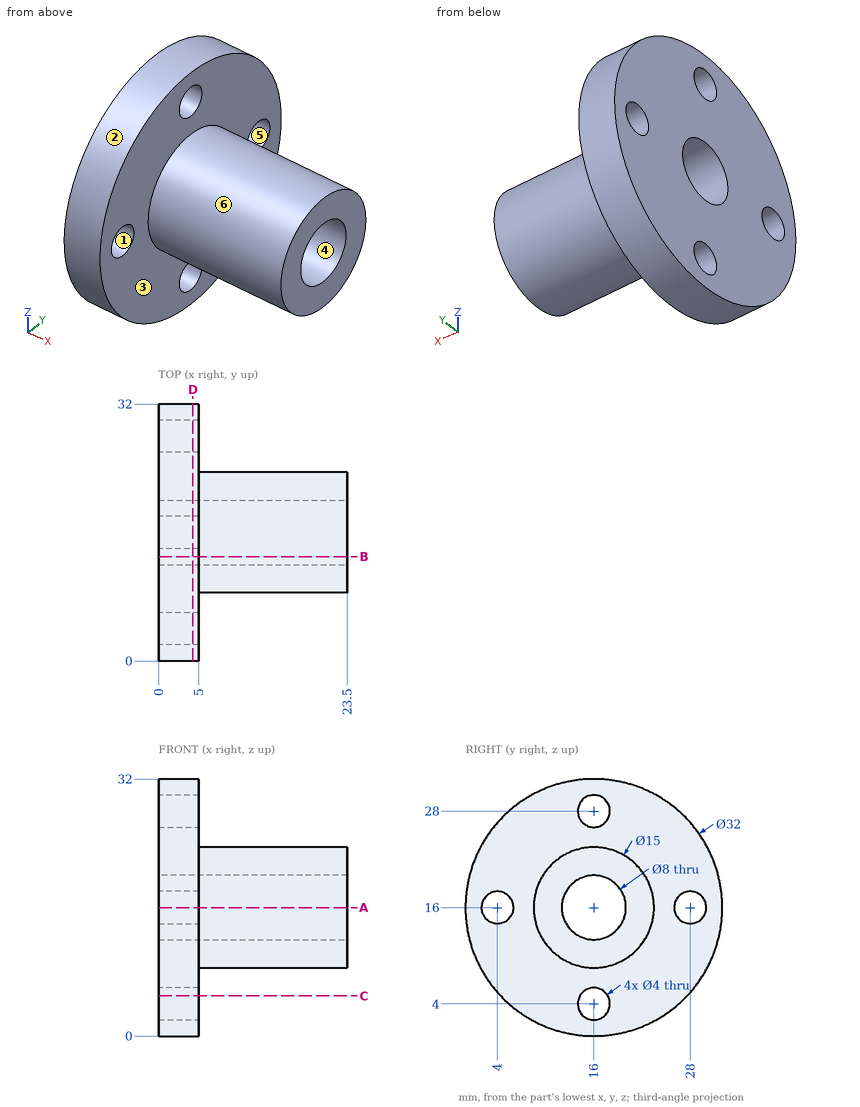
Could you check a few things on this drawing? It's one solid part, dimensions in mm from its lowest x, y, z. A direction names the side the tool comes from. Round coordinates to 2 decimals unless told otherwise and drop trailing zeros. Write each loop counter-clockwise with the first axis right and the second up, starting at its lowest first coordinate (ties: lowest second). Pieces come first, ordered by that corner, then holes.
Q1. Will these pins go through, and if not, where does the flat tip stop? P1, Ø5, axis at x = 2.5, z = 25.5, coming from the +Y side; P2, Ø4.5, axis at y = 28, z = 16, coming from the +X side; P3, Ø2, axis at x = 8.5, y = 18, coming from the -Z side; P4, Ø3.5, axis at y = 16, z = 28, coming from the -X side.
Q2. If we mould it in two halves opening along Y, with no side actions, what happens to the marked faces 1, 2, 3 and 4? For each: +Y half, -Y half, draft (parallel to the pull), parting line (faces both ways), or undercut.
Q3. If we section it at A-A on z = 16: Write out the boundary of the cut face in (x, y).
Q4. If we section it at C-C on z = 5: Write out the boundary of the cut face in (x, y), plus the area to 3 significant figures.
Q5. Which directions (+Z, -Z, +X, -X, +Y, -Y) give clear straight access to the entire face, cutting with the end or side of a thin tool? Please do the marked faces 5 and 6.
Q6. Please list where these lines run through material, in increasing order: probe 1 along Y at (x, z) = (3.3, 16); probe 2 along X at (y, z) = (25.5, 10); probe 3 along Y at (x, z) = (1.5, 13).
Q7. If we section it at D-D on x = 4.25: Write out the boundary of the cut face in (y, z).
Q8. If we section it at B-B on y = 13: Write out the boundary of the cut face in (x, z), plus the area to 3 significant figures.
Answer below:
1. P1: stops at y = 30.39
1. P2: stops at x = 5
1. P3: stops at z = 8.57
1. P4: passes through
2. face 1: undercut
2. face 2: parting line
2. face 3: draft
2. face 4: undercut
3. outline: (0, 0) - (5, 0) - (5, 2) - (0, 2) - close; (0, 6) - (5, 6) - (5, 8.5) - (23.5, 8.5) - (23.5, 12) - (0, 12) - close; (0, 20) - (23.5, 20) - (23.5, 23.5) - (5, 23.5) - (5, 26) - (0, 26) - close; (0, 30) - (5, 30) - (5, 32) - (0, 32) - close
4. outline: (0, 4.38) - (5, 4.38) - (5, 14.27) - (0, 14.27) - close; (0, 17.73) - (5, 17.73) - (5, 27.62) - (0, 27.62) - close
4. area: 98.9 mm2
5. face 5: +X, -X
5. face 6: +X
6. probe 1: y = 0 to 2, 6 to 12, 20 to 26, 30 to 32
6. probe 2: x = 0 to 5
6. probe 3: y = 0.28 to 13.35, 18.65 to 31.72
7. outline: circle Ø32 at (16, 16); hole circle Ø4 at (4, 16); hole circle Ø8 at (16, 16); hole circle Ø4 at (16, 4); hole circle Ø4 at (16, 28); hole circle Ø4 at (28, 16)
8. outline: (0, 0.28) - (5, 0.28) - (5, 9.13) - (23.5, 9.13) - (23.5, 13.35) - (0, 13.35) - close; (0, 18.65) - (23.5, 18.65) - (23.5, 22.87) - (5, 22.87) - (5, 31.72) - (0, 31.72) - close
8. area: 287 mm2
